from build123d import *

# Parameters (mm, degrees)
SKETCH3_W           = 3.68
SKETCH3_H           = 3.68
BOSS_EXTRUDE1_DEPTH = 1219.2


with BuildPart() as part:
    # Sketch3 → Boss-Extrude1 (new, symmetric)
    with BuildSketch(Plane.XY):
        with BuildLine():
            Line((-4.203948776, 6), (0, 6))
            Line((0, 6), (4.203948776, 6))
            Line((4.203948776, 6), (8.2, 9.996051224))
            Line((8.2, 9.996051224), (8.2, 12.71))
            Line((8.2, 12.71), (4, 12.71))
            Line((4, 12.71), (4, 14.5))
            Line((4, 14.5), (4.5, 14.5))
            Line((4.5, 14.5), (4.5, 15))
            Line((4.5, 15), (12.968, 15))
            ThreePointArc((12.968, 15), (14.404840979, 14.404840979), (15, 12.968))
            Line((15, 12.968), (15, 4.5))
            Line((15, 4.5), (14.5, 4.5))
            Line((14.5, 4.5), (14.5, 4))
            Line((14.5, 4), (12.71, 4))
            Line((12.71, 4), (12.71, 8.2))
            Line((12.71, 8.2), (9.996051224, 8.2))
            Line((9.996051224, 8.2), (6, 4.203948776))
            Line((6, 4.203948776), (6, 0))
            Line((6, 0), (6, -4.203948776))
            Line((6, -4.203948776), (9.996051224, -8.2))
            Line((9.996051224, -8.2), (12.71, -8.2))
            Line((12.71, -8.2), (12.71, -4))
            Line((12.71, -4), (14.5, -4))
            Line((14.5, -4), (14.5, -4.5))
            Line((14.5, -4.5), (15, -4.5))
            Line((15, -4.5), (15, -12.968))
            ThreePointArc((15, -12.968), (14.404840979, -14.404840979), (12.968, -15))
            Line((12.968, -15), (4.5, -15))
            Line((4.5, -15), (4.5, -14.5))
            Line((4.5, -14.5), (4, -14.5))
            Line((4, -14.5), (4, -12.71))
            Line((4, -12.71), (8.2, -12.71))
            Line((8.2, -12.71), (8.2, -9.996051224))
            Line((8.2, -9.996051224), (4.203948776, -6))
            Line((4.203948776, -6), (0, -6))
            Line((0, -6), (-4.203948776, -6))
            Line((-4.203948776, -6), (-8.2, -9.996051224))
            Line((-8.2, -9.996051224), (-8.2, -12.71))
            Line((-8.2, -12.71), (-4, -12.71))
            Line((-4, -12.71), (-4, -14.5))
            Line((-4, -14.5), (-4.5, -14.5))
            Line((-4.5, -14.5), (-4.5, -15))
            Line((-4.5, -15), (-12.968, -15))
            ThreePointArc((-12.968, -15), (-14.404840979, -14.404840979), (-15, -12.968))
            Line((-15, -12.968), (-15, -4.5))
            Line((-15, -4.5), (-14.5, -4.5))
            Line((-14.5, -4.5), (-14.5, -4))
            Line((-14.5, -4), (-12.71, -4))
            Line((-12.71, -4), (-12.71, -8.2))
            Line((-12.71, -8.2), (-9.996051224, -8.2))
            Line((-9.996051224, -8.2), (-6, -4.203948776))
            Line((-6, -4.203948776), (-6, 0))
            Line((-6, 0), (-6, 4.203948776))
            Line((-6, 4.203948776), (-9.996051224, 8.2))
            Line((-9.996051224, 8.2), (-12.71, 8.2))
            Line((-12.71, 8.2), (-12.71, 4))
            Line((-12.71, 4), (-14.5, 4))
            Line((-14.5, 4), (-14.5, 4.5))
            Line((-14.5, 4.5), (-15, 4.5))
            Line((-15, 4.5), (-15, 12.968))
            ThreePointArc((-15, 12.968), (-14.404840979, 14.404840979), (-12.968, 15))
            Line((-12.968, 15), (-4.5, 15))
            Line((-4.5, 15), (-4.5, 14.5))
            Line((-4.5, 14.5), (-4, 14.5))
            Line((-4, 14.5), (-4, 12.71))
            Line((-4, 12.71), (-8.2, 12.71))
            Line((-8.2, 12.71), (-8.2, 9.996051224))
            Line((-8.2, 9.996051224), (-4.203948776, 6))
        make_face()
        with Locations((-11.63, 11.63)):
            Rectangle(SKETCH3_W, SKETCH3_H, mode=Mode.SUBTRACT)
        with BuildLine():
            Line((-3.143089642, 4.493663594), (-1.705676589, 3.056250541))
            ThreePointArc((-1.705676589, 3.056250541), (0, 3.5), (1.705676589, 3.056250541))
            Line((1.705676589, 3.056250541), (3.143089642, 4.493663594))
            Line((3.143089642, 4.493663594), (4.493663594, 3.143089642))
            Line((4.493663594, 3.143089642), (3.056250541, 1.705676589))
            ThreePointArc((3.056250541, 1.705676589), (3.5, 0), (3.056250541, -1.705676589))
            Line((3.056250541, -1.705676589), (4.493663594, -3.143089642))
            Line((4.493663594, -3.143089642), (3.143089642, -4.493663594))
            Line((3.143089642, -4.493663594), (1.705676589, -3.056250541))
            ThreePointArc((1.705676589, -3.056250541), (0, -3.5), (-1.705676589, -3.056250541))
            Line((-1.705676589, -3.056250541), (-3.143089642, -4.493663594))
            Line((-3.143089642, -4.493663594), (-4.493663594, -3.143089642))
            Line((-4.493663594, -3.143089642), (-3.056250541, -1.705676589))
            ThreePointArc((-3.056250541, -1.705676589), (-3.5, 0), (-3.056250541, 1.705676589))
            Line((-3.056250541, 1.705676589), (-4.493663594, 3.143089642))
            Line((-4.493663594, 3.143089642), (-3.143089642, 4.493663594))
        make_face(mode=Mode.SUBTRACT)
        with Locations((11.63, 11.63)):
            Rectangle(SKETCH3_W, SKETCH3_H, mode=Mode.SUBTRACT)
        with Locations((11.63, -11.63)):
            Rectangle(SKETCH3_W, SKETCH3_H, mode=Mode.SUBTRACT)
        with Locations((-11.63, -11.63)):
            Rectangle(SKETCH3_W, SKETCH3_H, mode=Mode.SUBTRACT)
    extrude(amount=BOSS_EXTRUDE1_DEPTH, both=True)


solid = part.part
Can you work these out from the model? Positions are in its coordinate system, mm. Round coordinates to 2 decimals unless told otherwise and drop trailing zeros. Answer in a Markdown table with one row per item.
(1) Please list where these lines run through material, in increasing order: L1, parallel to Y at x = -11.5, z = -1027; L2, parallel to Y at x = -13.25, z = 813. Write a range as from..to.
From the geometry:
| item | result |
|---|---|
| L1 | y = -15..-13.47, -9.79..-8.2, 8.2..9.79, 13.47..15 |
| L2 | y = -14.98..-13.47, -9.79..-4, 4..9.79, 13.47..14.98 |
(2) For P1, Ø3, axis at y = -1, z = 78, coming from the -X side; P2, Ø1.4, axis at y = -14, z = 435.5, coming from the -X side; P3, Ø1, axis at y = 1, z = -648.5, coming from the +X side, each with a flat end and sliding along its axis, tell me the tip position at first contact or that it passes through.
From the geometry:
| item | result |
|---|---|
| P1 | stops at x = -6 |
| P2 | stops at x = -14.97 |
| P3 | stops at x = 6 |
(3) Suppose I cut it at A-A, the plane z = 530.5. Count the separate pieces of the cut face and the enclosed holes in it, plus the area to 3 significant figures.
From the geometry:
| item | result |
|---|---|
| separate pieces | 1 |
| enclosed holes | 5 |
| area | 337 mm2 |
